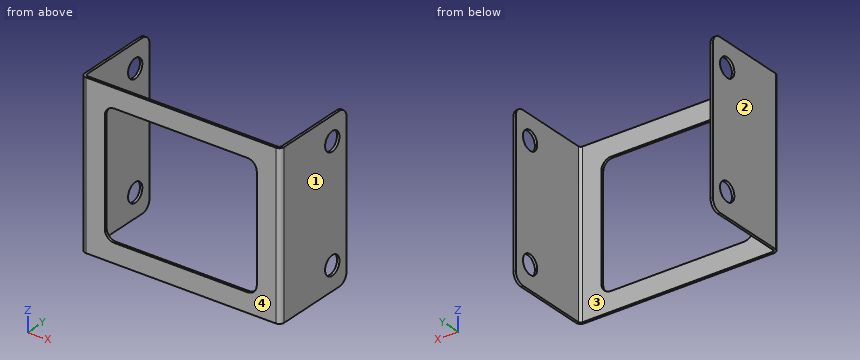
from build123d import *

# Parameters (mm, degrees)
SKETCH1_W          = 20
SKETCH1_H          = 17
BASE_FLANGE1_DEPTH = 0.25
CUT_EXTRUDE1_DEPTH = 14.126785593
EDGE_FLANGE2_DEPTH = 17
EDGE_FLANGE3_DEPTH = 17
FILLET1_R          = 1
SKETCH27_R         = 1
CUT_EXTRUDE2_DEPTH = 25.377243486


# Sheet-metal steps are written as plain solids
with BuildPart() as part:
    # Sketch1 → Base-Flange1 (new body)
    with BuildSketch(Plane(origin=(0, 0, 0), x_dir=(1, 0, 0), z_dir=(0, 1, 0))):
        Rectangle(SKETCH1_W, SKETCH1_H)
    extrude(amount=-BASE_FLANGE1_DEPTH)

    # Sketch6 → Cut-Extrude1 (cut, through all)
    with BuildSketch(Plane(origin=(0, 0, 0), x_dir=(1, 0, 0), z_dir=(0, 1, 0))):
        with BuildLine():
            Line((-7, 6.5), (7, 6.5))
            ThreePointArc((7, 6.5), (7.707106781, 6.207106781), (8, 5.5))
            Line((8, 5.5), (8, -5.5))
            ThreePointArc((8, -5.5), (7.707106781, -6.207106781), (7, -6.5))
            Line((7, -6.5), (-7, -6.5))
            ThreePointArc((-7, -6.5), (-7.707106781, -6.207106781), (-8, -5.5))
            Line((-8, -5.5), (-8, 5.5))
            ThreePointArc((-8, 5.5), (-7.707106781, 6.207106781), (-7, 6.5))
        make_face()
    extrude(amount=-CUT_EXTRUDE1_DEPTH, mode=Mode.SUBTRACT)

    # Edge-Flange2 section (across the edge) → Edge-Flange2 (add)
    with BuildSketch(Plane(origin=(10.25, 0, 8.5), x_dir=(-1, 0, 0), z_dir=(0, 0, -1))):
        with BuildLine():
            Line((-0.25, 0.25), (-0.25, 9))
            Line((-0.25, 9), (0, 9))
            Line((0, 9), (0, 0.25))
            ThreePointArc((0, 0.25), (0.073223305, 0.073223305), (0.25, 0))
            Line((0.25, 0), (0.25, -0.25))
            ThreePointArc((0.25, -0.25), (-0.103553391, -0.103553391), (-0.25, 0.25))
        make_face()
    extrude(amount=EDGE_FLANGE2_DEPTH)

    # Edge-Flange3 section (across the edge) → Edge-Flange3 (add)
    with BuildSketch(Plane(origin=(-10.25, 0, -8.5), x_dir=(1, 0, 0), z_dir=(0, 0, 1))):
        with BuildLine():
            Line((-0.25, 0.25), (-0.25, 9))
            Line((-0.25, 9), (0, 9))
            Line((0, 9), (0, 0.25))
            ThreePointArc((0, 0.25), (0.073223305, 0.073223305), (0.25, 0))
            Line((0.25, 0), (0.25, -0.25))
            ThreePointArc((0.25, -0.25), (-0.103553391, -0.103553391), (-0.25, 0.25))
        make_face()
    extrude(amount=EDGE_FLANGE3_DEPTH)

    # Fillet1
    fillet1_edges = [part.edges().sort_by_distance(p)[0] for p in [
        (10.375, 9, 8.5),
        (10.375, 9, -8.5),
        (-10.375, 9, -8.5),
        (-10.375, 9, 8.5),
    ]]
    fillet(fillet1_edges, radius=FILLET1_R)

    # Sketch27 → Cut-Extrude2 (cut, through all)
    with BuildSketch(Plane.ZY.offset(10.5)):
        with Locations(Location((-6, 7, 0), (0, 0, 270))):
            Circle(SKETCH27_R)
        with Locations(Location((6, 7, 0), (0, 0, 270))):
            Circle(SKETCH27_R)
    extrude(amount=-CUT_EXTRUDE2_DEPTH, mode=Mode.SUBTRACT)


solid = part.part
CAD build for the part. Positions are in the model's coordinates, mm. Face numbers are marked on the shaded views. Round coordinates to 2 decimals unless told otherwise and drop trailing zeros. Loops run counter-clockwise (first coordinate to the right, second up) from the corner with the lowest first, then second, coordinate; pieces in that order, holes last. Notation, with made-up numbers: M -24,83.25 L 15,83.25 A28 ccw 15,122.25 Z; hole C 49,88 d2. An arc over 180 degrees is marked long. One line per question, with ' | ' between items. Start each with the question number.
Item 1: Two-plate mould, pull along X, no slides. Class the marked faces 1, 2, 3 and 4: pulls with the +X half, pulls with the -X half, needs draft (parallel to the pull), parting line crosses it, or undercut.
Item 2: Cut at D-D, the plane y = 4.75. Write the cut outline in (x, z), plus the area to 3 significant figures.
Item 3: Wall check: line 1 (Z direction, x = -10.35, y = 7); line 2 (X direction, y = 5, z = 4.25); line 3 (Y direction, x = -8.5, z = -3.25). Give the ranges that are in metal, low to high.
Item 4: Cut at C-C, the plane z = 0.5. Write the cut outline in (x, y).
Item 5: Pin check, flat tips, straight feed: pin 1 Ø1.5 at (x, z) = (-8, 3.5) entering from +Y; pin 2 Ø1.8 at (y, z) = (7, 6) entering from +X. Stop position of each tip, or through.
Item 6: Cut at A-A, the plane y = 7. Write the cut outline in (x, z), plus the area to 3 significant figures.
Item 7: Cut at B-B, the plane x = 5. Write the cut outline in (y, z).
Responses:
1) face 1: pulls with the +X half | face 2: pulls with the -X half | face 3: undercut | face 4: needs draft
2) outline: M -10.5,-8.5 L -10.25,-8.5 L -10.25,8.5 L -10.5,8.5 Z; M 10.25,-8.5 L 10.5,-8.5 L 10.5,8.5 L 10.25,8.5 Z | area: 8.50 mm²
3) line 1: z = -8.5 to -7, -5 to 5, 7 to 8.5 | line 2: x = -10.5 to -10.25, 10.25 to 10.5 | line 3: y = -0.25 to 0
4) outline: M -10.5,0.25 A0.5 ccw -10,-0.25 L -8,-0.25 L -8,0 L -10,0 A0.25 cw -10.25,0.25 L -10.25,9 L -10.5,9 Z; M 8,-0.25 L 10,-0.25 A0.5 ccw 10.5,0.25 L 10.5,9 L 10.25,9 L 10.25,0.25 A0.25 cw 10,0 L 8,0 Z
5) pin 1: stops at y = 0 | pin 2: passes through
6) outline: M -10.5,-8.5 L -10.25,-8.5 L -10.25,-7 L -10.5,-7 Z; M -10.5,-5 L -10.25,-5 L -10.25,5 L -10.5,5 Z; M -10.5,7 L -10.25,7 L -10.25,8.5 L -10.5,8.5 Z; M 10.25,-8.5 L 10.5,-8.5 L 10.5,-7 L 10.25,-7 Z; M 10.25,-5 L 10.5,-5 L 10.5,5 L 10.25,5 Z; M 10.25,7 L 10.5,7 L 10.5,8.5 L 10.25,8.5 Z | area: 6.50 mm²
7) outline: M -0.25,-8.5 L 0,-8.5 L 0,-6.5 L -0.25,-6.5 Z; M -0.25,6.5 L 0,6.5 L 0,8.5 L -0.25,8.5 Z
